Part model, mm, in its own coordinate system. Face numbers are marked on the shaded views. A direction names the side the tool comes from. Round coordinates to 2 decimals unless told otherwise and drop trailing zeros. Loops run counter-clockwise (first coordinate to the right, second up) from the corner with the lowest first, then second, coordinate; pieces in that order, holes last. Notation, with made-up numbers: (31, -25) -> (81, -25) arc R29 cw to (81, 14) -> close; hole circle Ø3 at (83.25, -32.5). An arc over 180 degrees is marked (long way). Answer as CSV lines item,"result".
Autodesk Inventor part; units mm, degrees
ref_plane "YZ Plane" through (0, 0, 0) normal (1, 0, 0) x (0, 1, 0)
ref_plane "XZ Plane" through (0, 0, 0) normal (0, 1, 0) x (-1, 0, 0)
ref_plane "XY Plane" through (0, 0, 0) normal (0, 0, 1) x (1, 0, 0)
sketch "Skizze1" plane through (0, 0, 0) normal (0, 0, 1) x (1, 0, 0)
  line L0 (5, 19) -> (-5, 19)
  line L1 (-5, 19) -> (-5, -19)
  line L2 (-5, -19) -> (5, -19)
  line L3 (5, -19) -> (5, 19)
  line L4 (5, 19) -> (-5, -19) construction
  line L5 (-5, 19) -> (5, -19) construction
  point P0 (0, 0)
  dimension "d0" = 38
  dimension "d1" = 10
extrude "Extrusion1" add sketch "Skizze1" along normal blind 74
sketch "Skizze2" plane through (-5, -19, 0) normal (-1, 0, 0) x (0, 0, 1)
  line L0 (0, 38) -> (74, 38)
  line L1 (0, 38) -> (17, 38)
  line L2 (17, 38) -> (17, 18)
  line L3 (17, 18) -> (0, 18)
  line L4 (0, 18) -> (0, 38)
  line L5 (74, 38) -> (57, 38)
  line L6 (57, 38) -> (57, 18)
  line L7 (57, 18) -> (74, 18)
  line L8 (74, 18) -> (74, 38)
  line L9 (27, 38) -> (47, 38)
  line L10 (47, 38) -> (47, 18)
  line L11 (47, 18) -> (27, 18)
  line L12 (27, 18) -> (27, 38)
  line L13 (0, 0) -> (74, 0)
  point P0 (0, 19)
  dimension "d4" = 18
  dimension "d5" = 20
  dimension "d6" = 40
  dimension "d7" = 10
  dimension "d8" = 18
  dimension "d9" = 18
extrude "Extrusion2" cut sketch "Skizze2" against normal blind 74
fillet "Rundung1" radius 5 4 edges at (-5, 19, 22) (-5, 19, 52) (5, 19, 52) (5, 19, 22)
sketch "Skizze5" plane through (0, 0, 74) normal (0, 0, 1) x (1, 0, 0)
  line L0 (5, -19) -> (-5, -19)
  line L1 (-5, -19) -> (-5, -1)
  point P0 (0, 0)
  point P1 (0, -10)
  dimension "d33" = 9
  dimension "d34" = 5
hole "Bohrung3" at (0, -10, 74) direction (0, 0, -1) diameter 3.242 depth 14 tip angle 118
sketch "Skizze6" plane through (0, 0, 0) normal (0, 0, -1) x (-1, 0, 0)
  line L0 (5, -1) -> (5, -19)
  line L1 (5, -19) -> (-5, -19)
  point P0 (0, 0)
  point P1 (0, -10)
  dimension "d42" = 5
  dimension "d43" = 9
hole "Bohrung4" at (0, -10, 0) direction (0, 0, 1) diameter 3.242 depth 14 tip angle 118
sketch "Skizze7" plane through (5, -19, 74) normal (1, 0, 0) x (0, 0, -1)
  line L0 (74, 0) -> (0, 0)
  line L1 (0, 18) -> (0, 0)
  point P0 (74, 19)
  point P1 (37, 5)
  dimension "d51" = 5
  dimension "d52" = 37
hole "Bohrung5" at (5, -14, 37) direction (-1, 0, 0) diameter 3 end through all
sketch "Skizze8" plane through (-5, -1, 57) normal (0, 0, 1) x (1, 0, 0)
  line L0 (10, 0) -> (0, 0)
  line L1 (0, 0) -> (0, 15)
  point P0 (5, 1)
  point P1 (5, 12)
  dimension "d60" = 12
  dimension "d61" = 5
hole "Bohrung6" at (0, 11, 57) direction (0, 0, -1) diameter 4 end through all
properties part number "ABI_Führungsblock"
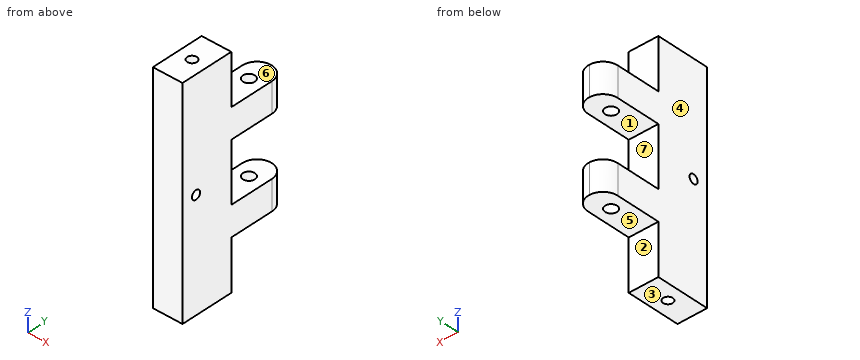
Q1. Saw through at C-C, the plane z = 37. Write the cut outline in (x, y).
Geometry results:
outline,"(-5, -19) -> (5, -19) -> (5, -15.5) -> (-5, -15.5) -> close; (-5, -12.5) -> (5, -12.5) -> (5, -1) -> (-5, -1) -> close"
Q2. Drop flat-ended pins along their axis: P1, Ø5, axis at x = -2, y = 7, coming from the +Z side; P2, Ø1.9, axis at x = 0, y = -10, coming from the -Z side; P3, Ø3, axis at x = -3.5, z = 26, coming from the +Y side. Give the stop position or say it passes through.
Geometry results:
P1,"z = 57"
P2,"z = 14.4"
P3,"y = 18.58"
Q3. Saw through at A-A, the plane y = -14. Write the cut outline in (x, z).
Geometry results:
outline,"(-5, 0) -> (5, 0) -> (5, 35.5) -> (-5, 35.5) -> close; (-5, 38.5) -> (5, 38.5) -> (5, 74) -> (-5, 74) -> close"
Q4. Saw through at D-D, the plane y = 11. Write the cut outline in (x, z).
Geometry results:
outline,"(-5, 17) -> (-2, 17) -> (-2, 27) -> (-5, 27) -> close; (-5, 47) -> (-2, 47) -> (-2, 57) -> (-5, 57) -> close; (2, 17) -> (5, 17) -> (5, 27) -> (2, 27) -> close; (2, 47) -> (5, 47) -> (5, 57) -> (2, 57) -> close"
Q5. Two-plate mould, pull along Z, no slides. Class the marked faces 1, 2 and 3: pulls with the +Z half, pulls with the -Z half, needs draft (parallel to the pull), parting line crosses it, or undercut.
Geometry results:
face 1,"undercut"
face 2,"needs draft"
face 3,"pulls with the -Z half"
Q6. Which spindle directions (+Z, -Z, +X, -X, +Y, -Y) get a long thin tool onto all of the face, cutting with end or side? Do the marked faces 4, 5, 6 and 7. Say none if no direction does.
Geometry results:
face 4,"+Z, -Z, -X, +Y, -Y"
face 5,"-Z, +X, -X, +Y"
face 6,"+Z, +X, -X, +Y"
face 7,"+X, -X, +Y"
Q7. Drill centre lines: line 1 along Y through (x, z) = (0, 69.75); line 2 along Z through (x, y) = (3.75, 7); line 3 along X through (y, z) = (11, 50). Where is each one in solid material? Low to high.
Geometry results:
line 1,"-19 to -11.62, -8.38 to -1"
line 2,"17 to 27, 47 to 57"
line 3,"-5 to -2, 2 to 5"
